Check sheet for the drawn part. Datum: minimum x, y, z corner. Units: mm. A direction names the side the tool comes from. Give positions to 0.01 mm unless a question says otherwise; leave off trailing zeros. Order: outer loops, then holes, each group sorted by start corner. A loop starts at its lowest first (then second) coordinate and runs counter-clockwise, first axis right, second up. Notation, with made-up numbers: (7.5, 22.5) -> (38.5, 22.5) arc R29 cw to (38.5, 43.5) -> close; hole circle Ø10 at (-33.5, -9). An arc over 180 degrees is marked (long way). One line per question, with ' | ' between items. Start each with the question number.
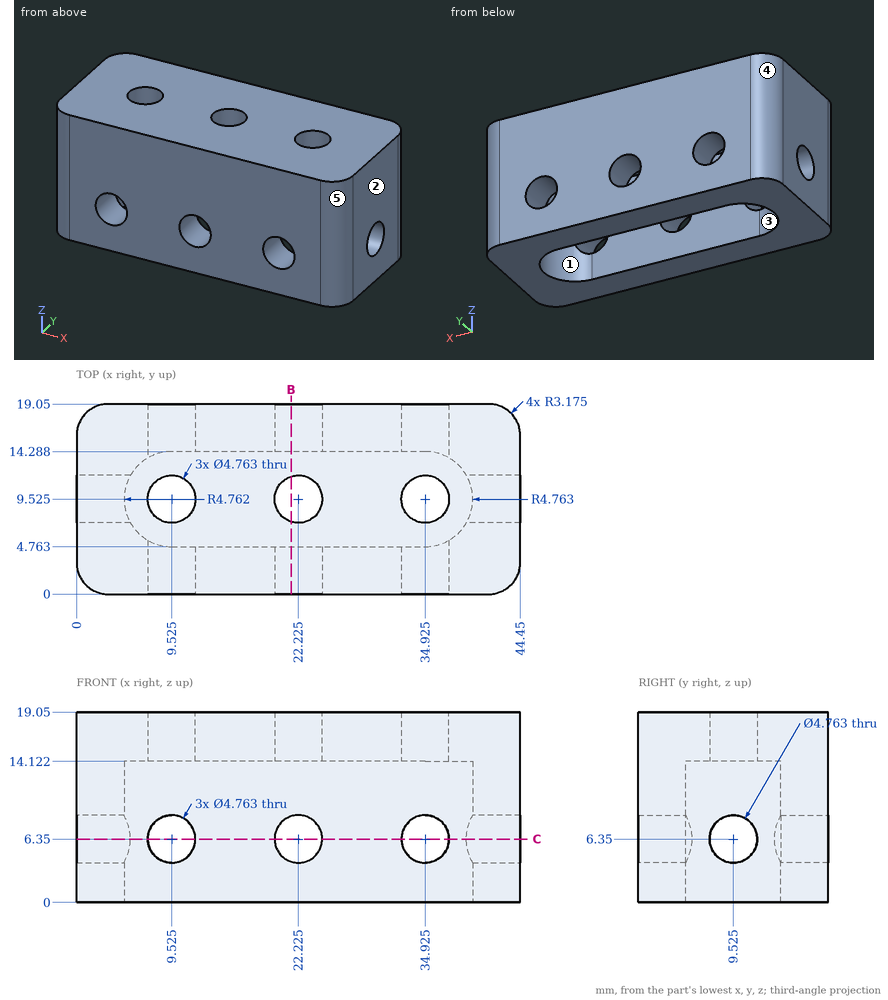
1. Cross-section at B-B on x = 21.5. Record the boundary of the cut face in (y, z).
2. Go/stop test with flat-tipped pins: pin 1 (6 mm diameter, centred on x = 22.225, z = 6.35, fed in from +Y); pin 2 (6 mm diameter, centred on x = 22.225, y = 9.525, fed in from -Z); pin 3 (4.5 mm diameter, centred on x = 9.525, z = 6.35, fed in from -Y). Record where each tip stops, or that it passes through.
3. Cross-section at C-C on z = 6.35. Give the number of separate pieces and of enclosed holes in the cut face.
4. Scan lines: probe 1 along Y at (x, z) = (19, 1.75); probe 2 along X at (y, z) = (2, 6.35) (1 decimal); probe 3 along X at (y, z) = (16.15, 6.35). Record each from-to range of solid material in increasing order.
5. Tool access check on the marked faces 1 and 2. Record the directions out of +Z, -Z, +X, -X, +Y, -Y that give a thin tool (end or side, any length) a straight path to the whole face; none if there is none.
6. Mould release check, pull along Y, two halves, no side actions. Record for the marked faces 3, 4 and 5: +Y half, -Y half, draft (parallel to the pull), parting line (faces both ways), or undercut.
Response values:
1) outline: (0, 0) -> (4.76, 0) -> (4.76, 4.08) -> (0, 4.08) -> close; (0, 8.62) -> (4.76, 8.62) -> (4.76, 14.12) -> (7.26, 14.12) -> (7.26, 19.05) -> (0, 19.05) -> close; (11.79, 14.12) -> (14.29, 14.12) -> (14.29, 8.62) -> (19.05, 8.62) -> (19.05, 19.05) -> (11.79, 19.05) -> close; (14.29, 0) -> (19.05, 0) -> (19.05, 4.08) -> (14.29, 4.08) -> close
2) pin 1: stops at y = 19.05 | pin 2: stops at z = 14.12 | pin 3: passes through
3) separate pieces: 8 | enclosed holes: 0
4) probe 1: y = 0 to 4.76, 14.29 to 19.05 | probe 2: x = 0.2 to 7.1, 11.9 to 19.8, 24.6 to 32.5, 37.3 to 44.2 | probe 3: x = 0.01 to 7.14, 11.91 to 19.84, 24.61 to 32.54, 37.31 to 44.44
5) face 1: -Z | face 2: +Z, -Z, +X, +Y, -Y
6) face 3: undercut | face 4: +Y half | face 5: -Y half
